Autodesk Inventor part; units mm, degrees
ref_plane "YZ Plane" through (0, 0, 0) normal (1, 0, 0) x (0, 1, 0)
ref_plane "XZ Plane" through (0, 0, 0) normal (0, 1, 0) x (-1, 0, 0)
ref_plane "XY Plane" through (0, 0, 0) normal (0, 0, 1) x (1, 0, 0)
sketch "Sketch2" plane through (0, 0, 0) normal (0, 1, 0) x (-1, 0, 0)
  line L0 (0, 0) -> (15.6172, 15.6172) construction
  line L1 (0, 0) -> (0, -11.6637) construction
  line L2 (-18.4102, -9.9249) -> (9.458, 17.9433) construction
  line L3 (0, 0) -> (8, 8)
  line L4 (8, 4.4645) -> (8, 4.4645)
  line L5 (8, 8) -> (8, 4.4645)
  line L6 (0, 0) -> (0, -3.5355)
  line L7 (0, 8.4853) -> (0, 12.0208)
  line L8 (0, 12.0208) -> (8, 20.0208)
  line L9 (8, 20.0208) -> (8, 16.4853)
  line L10 (0, 8.4853) -> (8, 16.4853)
  line L11 (8, 4.4645) -> (0, -3.5355)
  point P0 (-12.2426, -3.7574)
  dimension "d0" = 135
  dimension "d1" = 6
  dimension "d2" = 2.5
  dimension "d4" = 8
extrude "Extrusion1" add sketch "Sketch2" along normal blind 18
sketch "Sketch3" plane through (0, 0, 0) normal (0, -1, 0) x (1, 0, 0)
  line L0 (-8, 20.0208) -> (0, 12.0208)
  line L1 (-8, 4.4645) -> (0, -3.5355)
  line L2 (-8, 8) -> (-8, 4.4645)
  line L3 (0, 26.3321) -> (0, -17.8468)
  line L4 (-8, 16.4853) -> (-8, 20.0208)
  line L5 (0, 12.0208) -> (0, -3.5355)
  line L6 (-8, 4.4645) -> (-8, 20.0208)
  line L7 (-8, 20.0208) -> (0, 12.0208)
  line L8 (0, -3.5355) -> (-8, 4.4645)
  point P0 (0, 0)
extrude "Extrusion2" add sketch "Sketch3" along normal blind 2.5
sketch "Sketch4" plane through (0, 0, 0) normal (0, 0, 1) x (1, 0, 0)
  line L0 (-8, 18) -> (0, 18)
  line L1 (-2, 16) -> (-6, 16)
  line L2 (-6, 16) -> (-6, 12)
  line L3 (-6, 12) -> (-2, 12)
  line L4 (-2, 12) -> (-2, 16)
  line L5 (-4, 18) -> (-4, 0)
  line L6 (0, 0) -> (-8, 0)
  point P0 (-4, 16)
  dimension "d9" = 4
  dimension "d10" = 4
  dimension "d14" = 12
extrude "Extrusion3" cut sketch "Sketch4" along normal through all both and the other way through all
sketch "Sketch6" plane through (0, 0, 0) normal (0, 0, 1) x (1, 0, 0)
  line L0 (-2, 12) -> (-6, 12)
  line L1 (-4, 12) -> (-4, 2.9314) construction
  circle A0 centre (-4, 6.75) radius 0.75
  line L2 (0, 0) -> (-8, 0)
  dimension "d20" = 1.5
  dimension "d21" = 6
extrude "Extrusion5" cut sketch "Sketch6" along normal through all both and the other way through all
properties part number "gimbal_stick_fixation_big"
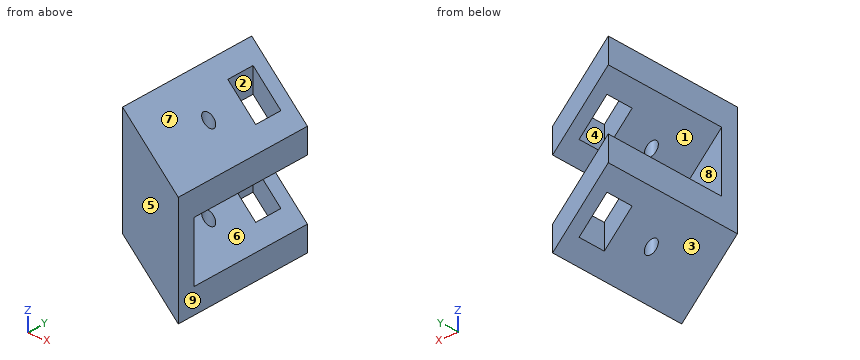
Here's how the part is built. I have some questions about the finished solid (model axes, mm). Face numbers are marked on the shaded views. A direction names the side the tool comes from. Coordinates: 2 decimals unless noted, no trailing zeros. Order: outer loops, then holes, each group sorted by start corner. A loop starts at its lowest first (then second) coordinate and runs counter-clockwise, first axis right, second up.
1) I need wall thicknesses on line 1 (Y direction, x = -4, z = 14.3); line 2 (Z direction, x = -6, y = 0.5); line 3 (Y direction, x = -4.5, z = 15). Which ranges of each line are inside material? Lowest first, please.
2) Which directions (+Z, -Z, +X, -X, +Y, -Y) give clear straight access to the entire face, cutting with the end or side of a thin tool? Please do the marked faces 1, 2, 3, 4 and 5.
3) Imagine slicing it at A-A on y = 1.25. List the corners of the cut face in (x, z) for me.
4) We'd pull the mould along Z, two halves only. Please class the marked faces 6, 7, 8 and 9: +Z half, -Z half, draft (parallel to the pull), parting line (faces both ways), or undercut.
5) Imagine slicing it at D-D on x = -4. List the corners of the cut face in (y, z) for me, and give its area (3 significant figures).
6) Imagine slicing it at B-B on y = 15. List the corners of the cut face in (x, z) for me, and give its area (3 significant figures).
7) Imagine slicing it at C-C on x = -2.5. List the corners of the cut face in (y, z) for me.
8) Will these pins go through, and if not, where does the flat tip stop? pin 1 (1 mm diameter, centred on x = -4.5, y = 9, fed in from -Z); pin 2 (1.1 mm diameter, centred on y = 14.5, z = -0.5, fed in from -X); pin 3 (1.7 mm diameter, centred on x = -4, y = 6.75, fed in from -Z).
Response values:
1. line 1: y = -2.5 to 6, 7.5 to 12, 16 to 18
1. line 2: z = 2.46 to 6, 14.49 to 18.02
1. line 3: y = -2.5 to 6.19, 7.31 to 12, 16 to 18
2. face 1: -X, +Y
2. face 2: +Z, -Z, +X
2. face 3: -Z, -X, +Y, -Y
2. face 4: +Z, -Z, -X
2. face 5: +Z, -Z, +X, -X, -Y
3. outline: (-8, 4.46) - (0, -3.54) - (0, 0) - (-8, 8) - close; (-8, 16.49) - (0, 8.49) - (0, 12.02) - (-8, 20.02) - close
4. face 6: undercut
4. face 7: +Z half
4. face 8: undercut
4. face 9: draft
5. outline: (-2.5, 0.46) - (6, 0.46) - (6, 4) - (0, 4) - (0, 12.49) - (6, 12.49) - (6, 16.02) - (-2.5, 16.02) - close; (7.5, 0.46) - (12, 0.46) - (12, 4) - (7.5, 4) - close; (7.5, 12.49) - (12, 12.49) - (12, 16.02) - (7.5, 16.02) - close; (16, 0.46) - (18, 0.46) - (18, 4) - (16, 4) - close; (16, 12.49) - (18, 12.49) - (18, 16.02) - (16, 16.02) - close
5. area: 127 mm2
6. outline: (-8, 4.46) - (-6, 2.46) - (-6, 6) - (-8, 8) - close; (-8, 16.49) - (-6, 14.49) - (-6, 18.02) - (-8, 20.02) - close; (-2, -1.54) - (0, -3.54) - (0, 0) - (-2, 2) - close; (-2, 10.49) - (0, 8.49) - (0, 12.02) - (-2, 14.02) - close
6. area: 28.3 mm2
7. outline: (-2.5, -1.04) - (12, -1.04) - (12, 2.5) - (0, 2.5) - (0, 10.99) - (12, 10.99) - (12, 14.52) - (-2.5, 14.52) - close; (16, -1.04) - (18, -1.04) - (18, 2.5) - (16, 2.5) - close; (16, 10.99) - (18, 10.99) - (18, 14.52) - (16, 14.52) - close
8. pin 1: stops at z = 0.46
8. pin 2: stops at x = -2
8. pin 3: stops at z = -0.39
